Input: part model. Units: mm. Frame: model coordinates. A direction names the side the tool comes from. Coordinates: 2 decimals unless noted, no trailing zeros. Order: outer loops, then holes, each group sorted by start corner. A loop starts at its lowest first (then second) coordinate and runs counter-clockwise, first axis right, second up. Notation, with made-up numbers: M -38.5,49.5 L 9.5,49.5 A6 cw 9.5,53.5 Z; hole C -30.5,-18 d2. An arc over 180 degrees is marked long. Answer in a Markdown table with one row per item.
from build123d import *

# Parameters (mm, degrees)
F0_R     = 4.1
F1_DEPTH = 6.5
F2_D     = 5.5
F3_R     = 5


with BuildPart() as f1:
    # F0 (on Top) → F1 (new body)
    with BuildSketch(Plane.XY):
        Polygon((18, 22), (0, 18), (0, 0), (0, -4), (18, 0), (38, 0), (38, 22), align=None)
        with Locations((6, 4)):
            Circle(F0_R, mode=Mode.SUBTRACT)
    extrude(amount=F1_DEPTH)

    # F2 (through all)
    with Locations(Plane(origin=(0, 0, 0), x_dir=(1, 0, 0), z_dir=(0, 0, -1))):
        with Locations((29.5, -17), (29.5, -5)):
            Hole(F2_D / 2)

    # F3
    f3_edges = [f1.edges().sort_by_distance(p)[0] for p in [
        (0, 18, 3.25),
        (0, -4, 3.25),
    ]]
    fillet(f3_edges, radius=F3_R)


solid = f1.part
1) Contact query for a flat-ended pin moving along its axis: pin 1 (2 mm diameter, centred on x = 6.5, z = 3, fed in from +Y). Output: stop coordinate, or through.
Resolved:
| item | result |
|---|---|
| pin 1 | stops at y = 19.67 |
2) Cut plane D-D, the plane y = 17. Output: boundary loops of the cut face in (x, z), and give its area (3 significant figures).
Resolved:
| item | result |
|---|---|
| outline | M 1.01,0 L 26.75,0 L 26.75,6.5 L 1.01,6.5 Z; M 32.25,0 L 38,0 L 38,6.5 L 32.25,6.5 Z |
| area | 205 mm2 |
3) Reachability of faces 5 (the face through (28, 0, 3)), 6 (the face through (38, 11, 3)) from +Z, -Z, +X, -X, +Y, -Y: full face, straight path, thin tool, end or side. Return the list, or none.
Resolved:
| item | result |
|---|---|
| face 5 | +Z, -Z, +X, -Y |
| face 6 | +Z, -Z, +X, +Y, -Y |
4) Cut plane A-A, the plane x = 29.5. Output: boundary loops of the cut face in (y, z).
Resolved:
| item | result |
|---|---|
| outline | M 0,0 L 2.25,0 L 2.25,6.5 L 0,6.5 Z; M 7.75,0 L 14.25,0 L 14.25,6.5 L 7.75,6.5 Z; M 19.75,0 L 22,0 L 22,6.5 L 19.75,6.5 Z |
5) Cut plane B-B, the plane y = 5.5. Output: boundary loops of the cut face in (x, z).
Resolved:
| item | result |
|---|---|
| outline | M 0,0 L 2.18,0 L 2.18,6.5 L 0,6.5 Z; M 9.82,0 L 26.8,0 L 26.8,6.5 L 9.82,6.5 Z; M 32.2,0 L 38,0 L 38,6.5 L 32.2,6.5 Z |
6) Cut plane C-C, the plane z = 4.5. Output: boundary loops of the cut face in (x, y).
Resolved:
| item | result |
|---|---|
| outline | M 0,2.23 A5 ccw 6.08,-2.65 L 18,0 L 38,0 L 38,22 L 18,22 L 3.92,18.87 A5 ccw 0,13.99 Z; hole C 6,4 d8.2; hole C 29.5,5 d5.5; hole C 29.5,17 d5.5 |
7) Material intervals for probe 1 along Y at (x, z) = (29.5, 2.5); probe 2 along X at (y, z) = (6.5, 5.5); probe 3 along X at (y, z) = (3.5, 2.25), sorted ascending.
Resolved:
| item | result |
|---|---|
| probe 1 | y = 0 to 2.25, 7.75 to 14.25, 19.75 to 22 |
| probe 2 | x = 0 to 2.75, 9.25 to 27.2, 31.8 to 38 |
| probe 3 | x = 0 to 1.93, 10.07 to 27.2, 31.8 to 38 |
8) Mould query, pull axis Y, two halves, no side actions, for faces 1 (the face through (19, 10, 6.5)), 2 (the face through (32.247, 4.879, 3.295)), 3 (the face through (9.787, 2.43, 3.204)), 4 (the face through (11.056, 20.457, 3.204)). Classes: +Y half, -Y half, draft (parallel to the pull), parting line (faces both ways), or undercut.
Resolved:
| item | result |
|---|---|
| face 1 | draft |
| face 2 | undercut |
| face 3 | undercut |
| face 4 | +Y half |
